from build123d import *

# Parameters (mm, degrees)
SKETCH1_W                      = 170
SKETCH1_H                      = 170
BOSS_EXTRUDE1_DEPTH            = 35
SKETCH2_W                      = 166
SKETCH2_H                      = 166
CUT_EXTRUDE1_DEPTH             = 33
SKETCH3_W                      = 2
SKETCH3_H                      = 170
BOSS_EXTRUDE2_DEPTH            = 15
SKETCH4_W                      = 2
SKETCH4_H                      = 170
BOSS_EXTRUDE3_DEPTH            = 15
F_3_0_3_DIAMETER_HOLE1_D       = 3
F_3_0_3_DIAMETER_HOLE1_DEPTH   = 100
F_3_0_3_DIAMETER_HOLE1_TIP     = 0.901290929
SKETCH7_R                      = 2.75
SKETCH7_W                      = 32
SKETCH7_H                      = 17
CUT_EXTRUDE2_DEPTH             = 15
FILLET1_R                      = 0.5
F_3_5_3_5_DIAMETER_HOLE1_D     = 3.5
F_3_5_3_5_DIAMETER_HOLE1_DEPTH = 100
F_3_5_3_5_DIAMETER_HOLE1_TIP   = 1.051506083


with BuildPart() as part:
    # Sketch1 → Boss-Extrude1 (new body)
    with BuildSketch(Plane.XY):
        Rectangle(SKETCH1_W, SKETCH1_H)
    extrude(amount=BOSS_EXTRUDE1_DEPTH)

    # Sketch2 → Cut-Extrude1 (cut)
    with BuildSketch(Plane.XY.offset(35)):
        Rectangle(SKETCH2_W, SKETCH2_H)
    extrude(amount=-CUT_EXTRUDE1_DEPTH, mode=Mode.SUBTRACT)

    # Sketch3 → Boss-Extrude2 (add)
    with BuildSketch(Plane(origin=(85, 0, 0), x_dir=(0, 0, -1), z_dir=(1, 0, 0))):
        with Locations((-34, 0)):
            Rectangle(SKETCH3_W, SKETCH3_H)
    extrude(amount=BOSS_EXTRUDE2_DEPTH)

    # Sketch4 → Boss-Extrude3 (add)
    with BuildSketch(Plane.ZY.offset(85)):
        with Locations((34, 0)):
            Rectangle(SKETCH4_W, SKETCH4_H)
    extrude(amount=BOSS_EXTRUDE3_DEPTH)

    # Ø3.0 (3) Diameter Hole1
    with Locations(Plane.XY.offset(35)):
        with Locations((-92.5, 45), (-92.5, -45), (115, -45), (115, 45), (92.5, 45), (92.5, -45)):
            Hole(F_3_0_3_DIAMETER_HOLE1_D / 2, depth=F_3_0_3_DIAMETER_HOLE1_DEPTH)
            with Locations((0, 0, -(F_3_0_3_DIAMETER_HOLE1_DEPTH + F_3_0_3_DIAMETER_HOLE1_TIP / 2))):  # 118° drill point
                Cone(0, F_3_0_3_DIAMETER_HOLE1_D / 2, F_3_0_3_DIAMETER_HOLE1_TIP, mode=Mode.SUBTRACT)

    # Sketch7 → Cut-Extrude2 (cut)
    with BuildSketch(Plane.XZ.offset(85)):
        with Locations((55, 15)):
            Circle(SKETCH7_R)
        with Locations((70, 15)):
            Circle(SKETCH7_R)
        with Locations((-34, 17.5)):
            Rectangle(SKETCH7_W, SKETCH7_H)
    extrude(amount=-CUT_EXTRUDE2_DEPTH, mode=Mode.SUBTRACT)

    # Fillet1
    fillet1_edges = [part.edges().sort_by_distance(p)[0] for p in [
        (-83, 0, 2),
        (83, 0, 2),
        (85, 0, 0),
        (85, 0, 33),
        (-85, 0, 0),
        (-85, 0, 33),
        (0, -85, 0),
        (0, 85, 0),
        (0, -83, 2),
    ]]
    fillet(fillet1_edges, radius=FILLET1_R)

    # Ø3.5 (3.5) Diameter Hole1
    with Locations(Plane.XZ.offset(85)):
        with Locations((-69, 28), (-1, 28), (-69, 18), (-1, 18), (-69, 8), (-1, 8)):
            Hole(F_3_5_3_5_DIAMETER_HOLE1_D / 2, depth=F_3_5_3_5_DIAMETER_HOLE1_DEPTH)
            with Locations((0, 0, -(F_3_5_3_5_DIAMETER_HOLE1_DEPTH + F_3_5_3_5_DIAMETER_HOLE1_TIP / 2))):  # 118° drill point
                Cone(0, F_3_5_3_5_DIAMETER_HOLE1_D / 2, F_3_5_3_5_DIAMETER_HOLE1_TIP, mode=Mode.SUBTRACT)


solid = part.part
Check sheet for the modelled part. Datum: model origin and axes. Units: mm. A direction names the side the tool comes from. Coordinates: 2 decimals unless noted, no trailing zeros. Write each loop counter-clockwise with the first axis right and the second up, starting at its lowest first coordinate (ties: lowest second). Pieces come first, ordered by that corner, then holes.
Item 1: Cross-section at B-B on x = 4. Record the boundary of the cut face in (y, z), then the cut area to 3 significant figures.
Numbers:
outline: (-85, 0.5) arc R0.5 ccw to (-84.5, 0) - (84.5, 0) arc R0.5 ccw to (85, 0.5) - (85, 35) - (83, 35) - (83, 2) - (-82.5, 2) arc R0.5 cw to (-83, 2.5) - (-83, 35) - (-85, 35) - close
area: 472 mm2
Item 2: Access from +Z, -Z, +X, -X, +Y, -Y to the whole of each face (thin tool, end or side, straight path). Record for faces 1 (the face through (-83, -1, 19)), 2 (the face through (85, -1, 16)), 3 (the face through (-93, -1, 33)), 4 (the face through (-88, -7, 35)), 5 (the face through (67.253, -84.014, 15.121)).
Numbers:
face 1: +Z
face 2: -Z, +X, +Y, -Y
face 3: -Z, -X, +Y, -Y
face 4: +Z, +X, -X, +Y, -Y
face 5: -Y
Item 3: Cross-section at A-A on x = 55. Record the boundary of the cut face in (y, z).
Numbers:
outline: (-85, 0.5) arc R0.5 ccw to (-84.5, 0) - (84.5, 0) arc R0.5 ccw to (85, 0.5) - (85, 35) - (83, 35) - (83, 2) - (-82.5, 2) arc R0.5 cw to (-83, 2.5) - (-83, 12.25) - (-85, 12.25) - close; (-85, 17.75) - (-83, 17.75) - (-83, 35) - (-85, 35) - close
Item 4: Cross-section at D-D on x = -36. Record the boundary of the cut face in (y, z).
Numbers:
outline: (-85, 0.5) arc R0.5 ccw to (-84.5, 0) - (84.5, 0) arc R0.5 ccw to (85, 0.5) - (85, 35) - (83, 35) - (83, 2) - (-82.5, 2) arc R0.5 cw to (-83, 2.5) - (-83, 9) - (-85, 9) - close; (-85, 26) - (-83, 26) - (-83, 35) - (-85, 35) - close
Item 5: Cross-section at C-C on y = 16.5. Record the boundary of the cut face in (x, z), then the cut area to 3 significant figures.
Numbers:
outline: (-100, 33) - (-85.5, 33) arc R0.5 cw to (-85, 32.5) - (-85, 0.5) arc R0.5 ccw to (-84.5, 0) - (84.5, 0) arc R0.5 ccw to (85, 0.5) - (85, 32.5) arc R0.5 cw to (85.5, 33) - (100, 33) - (100, 35) - (83, 35) - (83, 2.5) arc R0.5 cw to (82.5, 2) - (-82.5, 2) arc R0.5 cw to (-83, 2.5) - (-83, 35) - (-100, 35) - close
area: 532 mm2
Item 6: Mould release check, pull along Y, two halves, no side actions. Record for faces 6 (the face through (-85, -1, 16)), 7 (the face through (1, 85, 18)), 8 (the face through (83, -1, 19)): released by +Y, released by -Y, zero draft, split by the parting line, or undercut.
Numbers:
face 6: zero draft
face 7: released by +Y
face 8: undercut
Item 7: Scan lines: probe 1 along Z at (x, y) = (-69, -84.5); probe 2 along X at (y, z) = (68, 13). Record each from-to range of solid material in increasing order.
Numbers:
probe 1: z = 0 to 6.25, 9.75 to 16.25, 19.75 to 26.25, 29.75 to 35
probe 2: x = -85 to -83, 83 to 85
Item 8: Depth check by flat-ended pin: pin 1 Ø4 at (y, z) = (-29.5, 28) entering from -X; pin 2 Ø5 at (x, y) = (-92.5, 45) entering from +Z; pin 3 Ø4 at (x, y) = (-43, -9.5) entering from +Z; pin 4 Ø2 at (x, z) = (-1, 18) entering from -Y. Enter the tip coordinate at first touch or a pass-through.
Numbers:
pin 1: stops at x = -85
pin 2: stops at z = 35
pin 3: stops at z = 2
pin 4: stops at y = 83
